Build history of the part. All positions in model axes, mm. Face numbers are marked on the shaded views. Round coordinates to 2 decimals unless told otherwise and drop trailing zeros. Write each loop counter-clockwise with the first axis right and the second up, starting at its lowest first coordinate (ties: lowest second). Pieces come first, ordered by that corner, then holes. Notation, with made-up numbers: M 69,60 L 79,60 A19 cw 79,84 Z; hole C 82.25,26 d1. An arc over 180 degrees is marked long. Write item = value, one per line.
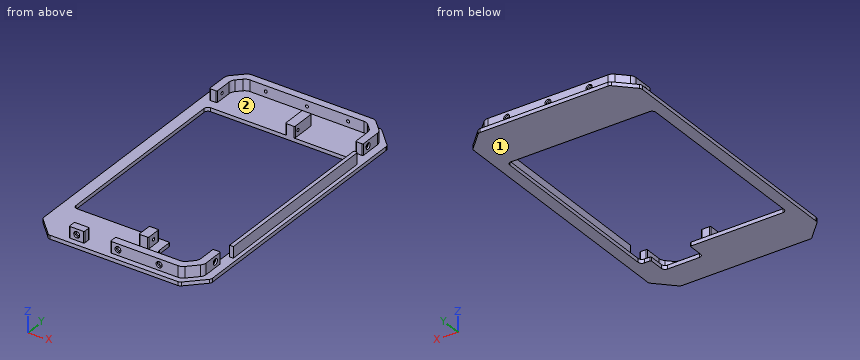
from build123d import *

# Parameters (mm, degrees)
SKETCH_1_W                = 90
SKETCH_1_H                = 156
EXTRUDE_1_DEPTH           = 2
CHAMFER_1_SIZE            = 10
EXTRUDE_2_DEPTH           = 6
SHELL_3_T                 = -4
SHELL_3_THICKNESS_2_DEPTH = 2
SKETCH_5_R                = 0.8
CUT_EXTRUDE_2088_DEPTH    = 200
SKETCH_25_W               = 15.521102544
SKETCH_25_H               = 165.941128128
SKETCH_25_W_2             = 34.04372952
CUT_EXTRUDE_17_DEPTH      = 6
SKETCH_8_W                = 109.527726605
SKETCH_8_H                = 110
CUT_EXTRUDE_3357_DEPTH    = 6
EXTRUDE_5_DEPTH           = 6
FILLET_4312_R             = 2
FILLET_4896_R             = 4
SKETCH_4_R                = 0.8
CUT_EXTRUDE_5906_DEPTH    = 100
SKETCH_6_W                = 5
SKETCH_6_H                = 13
SKETCH_6_H_2              = 8
EXTRUDE_3_DEPTH           = 6
CUT_EXTRUDE_START         = -10
SKETCH_17_R               = 0.8
CUT_EXTRUDE_7436_DEPTH    = 10
SKETCH_11_W               = 14
SKETCH_11_H               = 18.940292979
SKETCH_11_W_2             = 19
SKETCH_11_H_2             = 39.158001539
PCI_E_DEPTH               = 6
SKETCH_10_W               = 78
SKETCH_10_H               = 103
IO_2_DEPTH                = 10
SKETCH_15_W               = 21
SKETCH_15_H               = 10
CUT_EXTRUDE_10858_DEPTH   = 10
SKETCH_21_R               = 1.6
CUT_EXTRUDE_14_DEPTH      = 1
CUT_EXTRUDE_START_2       = -1
SKETCH_20_R               = 1.6
CUT_EXTRUDE_12604_DEPTH   = 1
SKETCH_22_R               = 1.6
CUT_EXTRUDE_15_DEPTH      = 1
SKETCH_23_R               = 1.6
CUT_EXTRUDE_16_DEPTH      = 1
SKETCH_26_W               = 2
SKETCH_26_H               = 96
EXTRUDE_4_DEPTH           = 6
FILLET_5_R                = 2
FILLET_7_R                = 0.5
FILLET_8_R                = 0.5


with BuildPart() as part:
    # 草图1 → 凸台-拉伸1 (new body)
    with BuildSketch(Plane.XY):
        with Locations((-45, 78)):
            Rectangle(SKETCH_1_W, SKETCH_1_H)
    extrude(amount=EXTRUDE_1_DEPTH)

    # 倒角1
    chamfer_1_edges = [part.edges().sort_by_distance(p)[0] for p in [
        (0, 0, 1),
        (-90, 0, 1),
        (-90, 156, 1),
        (0, 156, 1),
    ]]
    chamfer(chamfer_1_edges, length=CHAMFER_1_SIZE)

    # 草图2 → 凸台-拉伸2 (add)
    with BuildSketch(Plane.XY.offset(2)):
        Polygon((-78.757359313, 153), (-11.242640687, 153), (-3, 144.757359313), (-3, 11.242640687), (-11.242640687, 3), (-78.757359313, 3), (-87, 11.242640687), (-87, 144.757359313), align=None)
    extrude(amount=EXTRUDE_2_DEPTH)

    # 抽壳3
    shell_3_openings = [part.faces().sort_by_distance(p)[0] for p in [
        (-45, 78, 8),
    ]]
    offset(amount=SHELL_3_T, openings=shell_3_openings)

    # 抽壳3 thickness 2 face (on inner face of the shell) → 抽壳3 thickness 2 (cut)
    with BuildSketch(Plane(origin=(-45, 78, 4), x_dir=(-1, 0, 0), z_dir=(0, 0, -1))):
        Polygon((-32.100505063, 71), (32.100505063, 71), (38, 65.100505063), (38, -65.100505063), (32.100505063, -71), (-32.100505063, -71), (-38, -65.100505063), (-38, 65.100505063), align=None)
    extrude(amount=SHELL_3_THICKNESS_2_DEPTH, mode=Mode.SUBTRACT)

    # 草图5 → Cut-Extrude 2088 (cut)
    with BuildSketch(Plane(origin=(0, 3, 0), x_dir=(-1, 0, 0), z_dir=(0, -1, 0))):
        with Locations(Location((67, -5, 0), (0, 0, 90))):
            Circle(SKETCH_5_R)
        with Locations(Location((23, -5, 0), (0, 0, 90))):
            Circle(SKETCH_5_R)
        with Locations(Location((45, -5, 0), (0, 0, 90))):
            Circle(SKETCH_5_R)
    extrude(amount=-CUT_EXTRUDE_2088_DEPTH, mode=Mode.SUBTRACT)

    # 草图25 → 切除-拉伸17 (cut)
    with BuildSketch(Plane.XY.offset(8)):
        with Locations((-93.760551272, 70.734849479)):
            Rectangle(SKETCH_25_W, SKETCH_25_H)
        with Locations((13.02186476, 70.734849479)):
            Rectangle(SKETCH_25_W_2, SKETCH_25_H)
    extrude(amount=-CUT_EXTRUDE_17_DEPTH, mode=Mode.SUBTRACT)

    # 草图8 → Cut-Extrude 3357 (cut)
    with BuildSketch(Plane.XY.offset(8)):
        with Locations((-46.223461864, 78)):
            Rectangle(SKETCH_8_W, SKETCH_8_H)
    extrude(amount=-CUT_EXTRUDE_3357_DEPTH, mode=Mode.SUBTRACT)

    # 草图28 → 凸台-拉伸5 (add)
    with BuildSketch(Plane.XY.offset(2)):
        Polygon((-82, 143.100505063), (-82, 144.100505063), (-83, 143.100505063), (-83, 133), (-82, 133), align=None)
        Polygon((-8, 143.100505063), (-8, 144.100505063), (-7, 143.100505063), (-7, 133), (-8, 133), align=None)
        Polygon((-8, 12.899494937), (-8, 11.899494937), (-7, 12.899494937), (-7, 23), (-8, 23), align=None)
    extrude(amount=EXTRUDE_5_DEPTH)

    # Fillet 4312
    fillet_4312_edges = [part.edges().sort_by_distance(p)[0] for p in [
        (0, 146, 1),
        (0, 10, 1),
        (-80, 0, 1),
        (-10, 0, 1),
        (-90, 146, 1),
        (-90, 10, 1),
        (-10, 156, 1),
        (-80, 156, 1),
    ]]
    fillet(fillet_4312_edges, radius=FILLET_4312_R)

    # Fillet 4896
    fillet_4896_edges = [part.edges().sort_by_distance(p)[0] for p in [
        (-4, 145.757359313, 5),
        (-86, 10.242640687, 5),
        (-86, 145.757359313, 5),
        (-4, 10.242640687, 5),
        (-82, 144.100505063, 5),
        (-8, 144.100505063, 5),
        (-8, 11.899494937, 5),
        (-78.757359313, 153, 5),
        (-78.757359313, 3, 5),
        (-11.242640687, 3, 5),
        (-11.242640687, 153, 5),
        (-77.100505063, 149, 5),
        (-83, 12.899494937, 5),
        (-77.100505063, 7, 5),
        (-12.899494937, 7, 5),
        (-12.899494937, 149, 5),
    ]]
    fillet(fillet_4896_edges, radius=FILLET_4896_R)

    # 草图4 → Cut-Extrude 5906 (cut)
    with BuildSketch(Plane.ZY.offset(87)):
        with Locations(Location((5, 137, 0), (0, 0, 270))):
            Circle(SKETCH_4_R)
        with Locations(Location((5, 19, 0), (0, 0, 270))):
            Circle(SKETCH_4_R)
    extrude(amount=-CUT_EXTRUDE_5906_DEPTH, mode=Mode.SUBTRACT)

    # 草图6 → 凸台-拉伸3 (add)
    with BuildSketch(Plane.XY.offset(2)):
        with Locations((-39.5, 134.5)):
            Rectangle(SKETCH_6_W, SKETCH_6_H)
        with Locations((-39.5, 19)):
            Rectangle(SKETCH_6_W, SKETCH_6_H_2)
    extrude(amount=EXTRUDE_3_DEPTH)

    # 草图17 → Cut-Extrude 7436 (cut)
    with BuildSketch(Plane(origin=(-37, 0, 0), x_dir=(0, 0, -1), z_dir=(1, 0, 0)).offset(CUT_EXTRUDE_START)):
        with Locations((-5, 130.5)):
            Circle(SKETCH_17_R)
        with Locations(Location((-5, 19, 0), (0, 0, 270))):
            Circle(SKETCH_17_R)
    extrude(amount=CUT_EXTRUDE_7436_DEPTH, mode=Mode.SUBTRACT)

    # 草图11 → PCI-E (cut)
    with BuildSketch(Plane.XY.offset(8)):
        with Locations((-56, 6.415224672)):
            Rectangle(SKETCH_11_W, SKETCH_11_H)
        with Locations((-80.5, 14.172145087)):
            Rectangle(SKETCH_11_W_2, SKETCH_11_H_2)
    extrude(amount=-PCI_E_DEPTH, mode=Mode.SUBTRACT)

    # 草图10 → IO 2 (cut)
    with BuildSketch(Plane.XY.offset(8)):
        with Locations((-45, 76.5)):
            Rectangle(SKETCH_10_W, SKETCH_10_H)
    extrude(amount=-IO_2_DEPTH, mode=Mode.SUBTRACT)

    # 草图15 → Cut-Extrude 10858 (cut)
    with BuildSketch(Plane(origin=(0, 0, 0), x_dir=(-1, 0, 0), z_dir=(0, 0, -1))):
        with Locations((22, 20)):
            Rectangle(SKETCH_15_W, SKETCH_15_H)
    extrude(amount=-CUT_EXTRUDE_10858_DEPTH, mode=Mode.SUBTRACT)

    # 草图21 → 切除-拉伸14 (cut)
    with BuildSketch(Plane(origin=(0, 3, 0), x_dir=(-1, 0, 0), z_dir=(0, -1, 0))):
        with Locations(Location((67, -5, 0), (0, 0, 90))):
            Circle(SKETCH_21_R)
        with Locations(Location((45, -5, 0), (0, 0, 90))):
            Circle(SKETCH_21_R)
        with Locations(Location((23, -5, 0), (0, 0, 90))):
            Circle(SKETCH_21_R)
    extrude(amount=-CUT_EXTRUDE_14_DEPTH, mode=Mode.SUBTRACT)

    # 草图20 → Cut-Extrude 12604 (cut)
    with BuildSketch(Plane(origin=(0, 153, 0), x_dir=(1, 0, 0), z_dir=(0, 1, 0)).offset(CUT_EXTRUDE_START_2)):
        with Locations(Location((-67, -5, 0), (0, 0, 90))):
            Circle(SKETCH_20_R)
        with Locations(Location((-45, -5, 0), (0, 0, 90))):
            Circle(SKETCH_20_R)
        with Locations(Location((-23, -5, 0), (0, 0, 90))):
            Circle(SKETCH_20_R)
    extrude(amount=CUT_EXTRUDE_12604_DEPTH, mode=Mode.SUBTRACT)

    # 草图22 → 切除-拉伸15 (cut)
    with BuildSketch(Plane.ZY.offset(86)):
        with Locations(Location((5, 137, 0), (0, 0, 270))):
            Circle(SKETCH_22_R)
        with Locations((5, 19)):
            Circle(SKETCH_22_R)
    extrude(amount=-CUT_EXTRUDE_15_DEPTH, mode=Mode.SUBTRACT)

    # 草图23 → 切除-拉伸16 (cut)
    with BuildSketch(Plane(origin=(-4, 0, 0), x_dir=(0, 0, -1), z_dir=(1, 0, 0)).offset(CUT_EXTRUDE_START_2)):
        with Locations(Location((-5, 137, 0), (0, 0, 270))):
            Circle(SKETCH_23_R)
        with Locations(Location((-5, 19, 0), (0, 0, 90))):
            Circle(SKETCH_23_R)
    extrude(amount=CUT_EXTRUDE_16_DEPTH, mode=Mode.SUBTRACT)

    # 草图26 → 凸台-拉伸4 (add)
    with BuildSketch(Plane.XY.offset(2)):
        with Locations((-3, 78)):
            Rectangle(SKETCH_26_W, SKETCH_26_H)
    extrude(amount=EXTRUDE_4_DEPTH)

    # 圆角5
    fillet_5_edges = [part.edges().sort_by_distance(p)[0] for p in [
        (-84, 25, 1),
        (-6, 128, 1),
        (-6, 25, 1),
        (-84, 128, 1),
        (-11.5, 15, 1),
        (-32.5, 15, 1),
    ]]
    fillet(fillet_5_edges, radius=FILLET_5_R)

    # 圆角7
    fillet_7_edges = [part.edges().sort_by_distance(p)[0] for p in [
        (-32.5, 25, 1),
        (-11.5, 25, 1),
    ]]
    fillet(fillet_7_edges, radius=FILLET_7_R)

    # 圆角8
    fillet_8_edges = [part.edges().sort_by_distance(p)[0] for p in [
        (-86, 133, 5),
        (-4, 23, 5),
        (-4, 133, 5),
        (-82, 133, 5),
        (-8, 133, 5),
        (-8, 23, 5),
        (-42, 141, 5),
        (-42, 128, 5),
        (-37, 128, 5),
        (-37, 141, 5),
        (-37, 15, 5),
        (-37, 23, 5),
        (-42, 23, 5),
        (-42, 15, 5),
        (-49, 7, 5),
        (-63, 7, 5),
        (-71, 7, 5),
        (-71, 3, 5),
        (-63, 3, 5),
        (-49, 3, 5),
        (-4, 126, 5),
        (-2, 126, 5),
    ]]
    fillet(fillet_8_edges, radius=FILLET_8_R)


solid = part.part
1. Band-saw the part on A-A (y = 114.5). List the corners of the cut face in (x, z).
Responses:
outline = M -90,0 L -84,0 L -84,2 L -90,2 Z; M -6,0 L 0,0 L 0,2 L -2,2 L -2,8 L -4,8 L -4,2 L -6,2 Z
2. Band-saw the part on B-B (x = -54). List the corners of the cut face in (y, z).
Responses:
outline = M 0,0 L 25,0 L 25,2 L 0,2 Z; M 128,0 L 156,0 L 156,2 L 153,2 L 153,8 L 149,8 L 149,2 L 128,2 Z
3. Probe probe 1 along X at (y, z) = (139, 2.75); probe 2 along Y at (x, z) = (-64.5, 3.25); probe 3 along X at (y, z) = (55, 1.25). List the from-to ranges inside material, lowest first.
Responses:
probe_1 = -86 to -82, -42 to -37, -8 to -4
probe_2 = 3 to 7, 149 to 153
probe_3 = -90 to -84, -6 to 0
4. Mould opens along Y. For the marked faces 1 and 2 say: pulls with the +Y half, pulls with the -Y half, needs draft (parallel to the pull), parting line crosses it, or undercut.
Responses:
face_1 = needs draft
face_2 = undercut
5. Flat gauge pins, fed straight in: pin 1 (3.5 mm diameter, centred on x = -23, z = 5, fed in from +Y); pin 2 (8 mm diameter, centred on x = -68, y = 22.5, fed in from -Z); pin 3 (1.8 mm diameter, centred on y = 73, z = 6, fed in from +X); pin 4 (1.9 mm diameter, centred on x = -67, z = 5, fed in from +Y). Where does each tip first touch, or does it go through?
Responses:
pin_1 = 153
pin_2 = 0
pin_3 = -2
pin_4 = 152
